Source: CAD feature listing. Evaluate the final solid. Frame: model axes, mm. A direction names the side the tool comes from. Give positions to 0.01 mm unless a question says otherwise; leave off trailing zeros. Loops run counter-clockwise (first coordinate to the right, second up) from the corner with the lowest first, then second, coordinate; pieces in that order, holes last. Notation, with made-up numbers: (-6, 11.5) -> (33, 11.5) arc R21 cw to (33, 39.5) -> close; hole circle Ø1 at (28, -31). An arc over 180 degrees is marked (long way). Answer as a JSON object with one key per item and string values. Group by question number.
from build123d import *

# Parameters (mm, degrees)
SKETCH1_W           = 21
SKETCH1_H           = 50
SKETCH1_R           = 2.6
BOSS_EXTRUDE1_DEPTH = 8
SKETCH2_R           = 5.5
CUT_EXTRUDE1_DEPTH  = 5
BOSS_EXTRUDE2_DEPTH = 50
CUT_EXTRUDE2_REACH  = 5
SKETCH4_W           = 2
SKETCH4_H           = 5


with BuildPart() as part:
    # Sketch1 → Boss-Extrude1 (new body)
    with BuildSketch(Plane(origin=(0, 0, 0), x_dir=(1, 0, 0), z_dir=(0, 1, 0))):
        Rectangle(SKETCH1_W, SKETCH1_H)
        with Locations((0, -15)):
            Circle(SKETCH1_R, mode=Mode.SUBTRACT)
        Circle(SKETCH1_R, mode=Mode.SUBTRACT)
        with Locations((0, 15)):
            Circle(SKETCH1_R, mode=Mode.SUBTRACT)
    extrude(amount=BOSS_EXTRUDE1_DEPTH)

    # Sketch2 → Cut-Extrude1 (cut)
    with BuildSketch(Plane.XZ):
        Circle(SKETCH2_R)
        with Locations((0, 15)):
            Circle(SKETCH2_R)
        with Locations((0, -15)):
            Circle(SKETCH2_R)
    extrude(amount=-CUT_EXTRUDE1_DEPTH, mode=Mode.SUBTRACT)

    # Sketch3 → Boss-Extrude2 (add)
    with BuildSketch(Plane.XY.offset(25)):
        Polygon((10.5, 8), (10.5, 0), (26.5, 0), (26.5, 14.555402141), (23.5, 14.555402141), (23.5, 3), (13.5, 3), (13.5, 14.555402141), (10.5, 14.555402141), align=None)
    extrude(amount=-BOSS_EXTRUDE2_DEPTH)

    # Sketch4 → Cut-Extrude2 (cut, up to next)
    with BuildSketch(Plane(origin=(0, 3, 0), x_dir=(1, 0, 0), z_dir=(0, 1, 0)), mode=Mode.PRIVATE) as cut_extrude2_sk1:
        with Locations((14.5, -15.5)):
            Rectangle(SKETCH4_W, SKETCH4_H)
    cut_extrude2_tool1 = extrude(cut_extrude2_sk1.sketch, amount=-CUT_EXTRUDE2_REACH, mode=Mode.PRIVATE) & part.part
    add(cut_extrude2_tool1.solids().sort_by_distance((14.5, 3, 15.5))[0], mode=Mode.SUBTRACT)
    # Sketch4 → Cut-Extrude2 (cut, up to next)
    with BuildSketch(Plane(origin=(0, 3, 0), x_dir=(1, 0, 0), z_dir=(0, 1, 0)), mode=Mode.PRIVATE) as cut_extrude2_sk2:
        with Locations((14.5, 15.5)):
            Rectangle(SKETCH4_W, SKETCH4_H)
    cut_extrude2_tool2 = extrude(cut_extrude2_sk2.sketch, amount=-CUT_EXTRUDE2_REACH, mode=Mode.PRIVATE) & part.part
    add(cut_extrude2_tool2.solids().sort_by_distance((14.5, 3, -15.5))[0], mode=Mode.SUBTRACT)
    # Sketch4 → Cut-Extrude2 (cut, up to next)
    with BuildSketch(Plane(origin=(0, 3, 0), x_dir=(1, 0, 0), z_dir=(0, 1, 0)), mode=Mode.PRIVATE) as cut_extrude2_sk3:
        with Locations((22.5, 0)):
            Rectangle(SKETCH4_W, SKETCH4_H)
    cut_extrude2_tool3 = extrude(cut_extrude2_sk3.sketch, amount=-CUT_EXTRUDE2_REACH, mode=Mode.PRIVATE) & part.part
    add(cut_extrude2_tool3.solids().sort_by_distance((22.5, 3, 0))[0], mode=Mode.SUBTRACT)
    # Sketch4 → Cut-Extrude2 (cut, up to next)
    with BuildSketch(Plane(origin=(0, 3, 0), x_dir=(1, 0, 0), z_dir=(0, 1, 0)), mode=Mode.PRIVATE) as cut_extrude2_sk4:
        with Locations((14.5, 0)):
            Rectangle(SKETCH4_W, SKETCH4_H)
    cut_extrude2_tool4 = extrude(cut_extrude2_sk4.sketch, amount=-CUT_EXTRUDE2_REACH, mode=Mode.PRIVATE) & part.part
    add(cut_extrude2_tool4.solids().sort_by_distance((14.5, 3, 0))[0], mode=Mode.SUBTRACT)
    # Sketch4 → Cut-Extrude2 (cut, up to next)
    with BuildSketch(Plane(origin=(0, 3, 0), x_dir=(1, 0, 0), z_dir=(0, 1, 0)), mode=Mode.PRIVATE) as cut_extrude2_sk5:
        with Locations((22.5, 15.5)):
            Rectangle(SKETCH4_W, SKETCH4_H)
    cut_extrude2_tool5 = extrude(cut_extrude2_sk5.sketch, amount=-CUT_EXTRUDE2_REACH, mode=Mode.PRIVATE) & part.part
    add(cut_extrude2_tool5.solids().sort_by_distance((22.5, 3, -15.5))[0], mode=Mode.SUBTRACT)
    # Sketch4 → Cut-Extrude2 (cut, up to next)
    with BuildSketch(Plane(origin=(0, 3, 0), x_dir=(1, 0, 0), z_dir=(0, 1, 0)), mode=Mode.PRIVATE) as cut_extrude2_sk6:
        with Locations((22.5, -15.5)):
            Rectangle(SKETCH4_W, SKETCH4_H)
    cut_extrude2_tool6 = extrude(cut_extrude2_sk6.sketch, amount=-CUT_EXTRUDE2_REACH, mode=Mode.PRIVATE) & part.part
    add(cut_extrude2_tool6.solids().sort_by_distance((22.5, 3, 15.5))[0], mode=Mode.SUBTRACT)


solid = part.part
(1) Access query for faces 4 (the face through (-1.19, 2.46, -5.37)), 5 (the face through (22, 2, -2.5)), 6 (the face through (10.5, 11, 0)). Directions: +Z, -Z, +X, -X, +Y, -Y. A direction counts if a zero-diameter tool reaches every point of the face in a straight line with its end or side. Return the directions, or none.
(2) Section query B-B on x = 0. Return the cut outline in (y, z).
(3) Material intervals for line 1 (Z direction, x = 0, y = 1.6); line 2 (Z direction, x = 0, y = 6.85); line 3 (X direction, y = 5.75, z = 0), sorted ascending. Write a range as from..to.
(4) Mould query, pull axis Z, two halves, no side actions, for faces 1 (the face through (8, 6, 25)), 2 (the face through (-1.19, 2.46, 9.63)), 3 (the face through (26.5, 7, 0)). Classes: pulls with the +Z half, pulls with the -Z half, needs draft (parallel to the pull), parting line crosses it, or undercut.
(5) Section query A-A on y = 7. Return the cut outline in (x, z).
(6) Section query D-D on z = -15. Return the cut outline in (x, y), plus the area to 3 significant figures.
(7) Section query C-C on y = 10.75. Return the cut outline in (x, z).
(8) First-contact query: pin 1 (10.5 mm diameter, centred on x = 3, z = -10.5, fed in from +Y); pin 2 (9 mm diameter, centred on x = 0, z = 15, fed in from -Y); pin 3 (4.5 mm diameter, centred on x = 0, z = -15, fed in from +Y); pin 4 (3.5 mm diameter, centred on y = 11, z = -8.5, fed in from -X). Flat tips, straight axial feed; report the tip coordinate or a pass-through.
Result:
{
 "1": {"face 4": "-Y", "face 5": "+Y, -Y", "face 6": "+Z, -Z, -X, +Y"},
 "2": {"outline": "(0, -25) -> (8, -25) -> (8, -17.6) -> (5, -17.6) -> (5, -20.5) -> (0, -20.5) -> close; (0, -9.5) -> (5, -9.5) -> (5, -12.4) -> (8, -12.4) -> (8, -2.6) -> (5, -2.6) -> (5, -5.5) -> (0, -5.5) -> close; (0, 5.5) -> (5, 5.5) -> (5, 2.6) -> (8, 2.6) -> (8, 12.4) -> (5, 12.4) -> (5, 9.5) -> (0, 9.5) -> close; (0, 20.5) -> (5, 20.5) -> (5, 17.6) -> (8, 17.6) -> (8, 25) -> (0, 25) -> close"},
 "3": {"line 1": "-25..-20.5, -9.5..-5.5, 5.5..9.5, 20.5..25", "line 2": "-25..-17.6, -12.4..-2.6, 2.6..12.4, 17.6..25", "line 3": "-10.5..-2.6, 2.6..13.5, 23.5..26.5"},
 "4": {"face 1": "pulls with the +Z half", "face 2": "undercut", "face 3": "needs draft"},
 "5": {"outline": "(-10.5, -25) -> (13.5, -25) -> (13.5, 25) -> (-10.5, 25) -> close; (23.5, -25) -> (26.5, -25) -> (26.5, 25) -> (23.5, 25) -> close; hole circle Ø5.2 at (0, -15); hole circle Ø5.2 at (0, 0); hole circle Ø5.2 at (0, 15)"},
 "6": {"outline": "(-10.5, 0) -> (-5.5, 0) -> (-5.5, 5) -> (-2.6, 5) -> (-2.6, 8) -> (-10.5, 8) -> close; (2.6, 5) -> (5.5, 5) -> (5.5, 0) -> (13.5, 0) -> (13.5, 14.56) -> (10.5, 14.56) -> (10.5, 8) -> (2.6, 8) -> close; (15.5, 0) -> (21.5, 0) -> (21.5, 3) -> (15.5, 3) -> close; (23.5, 0) -> (26.5, 0) -> (26.5, 14.56) -> (23.5, 14.56) -> close", "area": "203 mm²"},
 "7": {"outline": "(10.5, -25) -> (13.5, -25) -> (13.5, 25) -> (10.5, 25) -> close; (23.5, -25) -> (26.5, -25) -> (26.5, 25) -> (23.5, 25) -> close"},
 "8": {"pin 1": "y = 8", "pin 2": "y = 5", "pin 3": "through", "pin 4": "x = 10.5"}
}
